Geometry check sheet. Reference: the model listing, model coordinates, mm. A direction names the side the tool comes from. Round coordinates to 2 decimals unless told otherwise and drop trailing zeros. Order: outer loops, then holes, each group sorted by start corner. A loop starts at its lowest first (then second) coordinate and runs counter-clockwise, first axis right, second up. Notation, with made-up numbers: (43, 52) -> (58, 52) arc R12 cw to (58, 64) -> close; hole circle Ø4 at (-1, 63). An arc over 180 degrees is marked (long way). Use a Markdown table: item, result. Add a question column.
Item 1: Sectioned sample at C-C, the plane z = 47. Record the cut outline in (x, y), and give its area (3 significant figures).
Item 2: Gauge pin test, flat ends, axial feed: pin 1 Ø4 at (x, z) = (-16.5, 75) entering from -Y; pin 2 Ø0.6 at (y, z) = (12.5, 202) entering from +X; pin 3 Ø10.5 at (y, z) = (19.5, 99) entering from +X; pin 4 Ø1.3 at (y, z) = (22.5, -2.5) entering from -X. Record the tip position at first contact, or that the pin passes through.
Item 3: Set-up check for faces 1 (the flat face through (-31, 22.103, -2)), 2 (the flat face through (-61.179, 17, 108)), 3 (the flat face through (-61, 23.303, 75)), 4 (the flat face through (-39, 1, 220)), 5 (the flat face through (-30, 13, 2)): record each of +Z, -Z, +X, -X, +Y, -Y from which the full face is reachable in a straight line by a thin tool's end or side.
Item 4: Sectioned sample at D-D, the plane y = 9. Record the cut outline in (x, z).
Item 5: Sectioned sample at B-B, the plane x = -35. Record the cut outline in (y, z), and give its area (3 significant figures).
Item 6: Material ranges on probe 1 along X at (y, z) = (13.5, 34.5); probe 2 along X at (y, z) = (21.75, 135.5); probe 3 along Z at (x, y) = (-13.5, 21.5), recorded low to high. Write a range as [from, to].
Item 7: Sectioned sample at A-A, the plane z = 149. Record the cut outline in (x, y).
from build123d import *

# Parameters (mm, degrees)
F1_DEPTH = 220
F3_DEPTH = 2
F5_DEPTH = 2
F6_W     = 61.179483
F6_H     = 1.2
F7_DEPTH = 5


with BuildPart() as f1:
    # F0 (on Top) → F1 (new body)
    with BuildSketch(Plane.XY):
        Polygon((-51.641022, 0), (0, 0), (0, 2), (-49.641022, 2), (-49.641022, 13.641025), (-59.179483, 13.641025), (-59.179483, 23.302566), (-63.948719, 23.302566), (-63.948719, 22.102566), (-61.179483, 22.102566), (-61.179483, 11.641025), (-51.641022, 11.641025), align=None)
    extrude(amount=F1_DEPTH)

    # F2 (on face) → F3 (cut, through all)
    with BuildSketch(Plane(origin=(0, 13.641025, 0), x_dir=(-1, 0, 0), z_dir=(0, 1, 0))):
        with BuildLine():
            Line((57.179483, 189.76923), (57.179483, 214.23077))
            ThreePointArc((57.179483, 214.23077), (54.410253, 217), (51.641022, 214.23077))
            Line((51.641022, 214.23077), (51.641022, 189.76923))
            ThreePointArc((51.641022, 189.76923), (54.410253, 187), (57.179483, 189.76923))
        make_face()
        with BuildLine():
            Line((57.179483, 144.76923), (57.179483, 169.23077))
            ThreePointArc((57.179483, 169.23077), (54.410253, 172), (51.641022, 169.23077))
            Line((51.641022, 169.23077), (51.641022, 144.76923))
            ThreePointArc((51.641022, 144.76923), (54.410253, 142), (57.179483, 144.76923))
        make_face()
        with BuildLine():
            Line((57.179483, 99.76923), (57.179483, 124.23077))
            ThreePointArc((57.179483, 124.23077), (54.410253, 127), (51.641022, 124.23077))
            Line((51.641022, 124.23077), (51.641022, 99.76923))
            ThreePointArc((51.641022, 99.76923), (54.410253, 97), (57.179483, 99.76923))
        make_face()
        with BuildLine():
            Line((57.179483, 54.76923), (57.179483, 79.23077))
            ThreePointArc((57.179483, 79.23077), (54.410253, 82), (51.641022, 79.23077))
            Line((51.641022, 79.23077), (51.641022, 54.76923))
            ThreePointArc((51.641022, 54.76923), (54.410253, 52), (57.179483, 54.76923))
        make_face()
        with BuildLine():
            Line((57.179483, 9.76923), (57.179483, 34.23077))
            ThreePointArc((57.179483, 34.23077), (54.410253, 37), (51.641022, 34.23077))
            Line((51.641022, 34.23077), (51.641022, 9.76923))
            ThreePointArc((51.641022, 9.76923), (54.410253, 7), (57.179483, 9.76923))
        make_face()
    extrude(amount=-F3_DEPTH, mode=Mode.SUBTRACT)

    # F4 (on face) → F5 (join)
    with BuildSketch(Plane(origin=(0, 0, 0), x_dir=(1, 0, 0), z_dir=(0, 0, -1))):
        Polygon((-59.179483, -13.641025), (-59.179483, -23.302566), (0, -23.302566), (0, -2), (-49.641022, -2), (-49.641022, -13.641025), align=None)
    extrude(amount=-F5_DEPTH)

    # F6 (on face) → F7 (join)
    with BuildSketch(Plane(origin=(0, 0, 0), x_dir=(1, 0, 0), z_dir=(0, 0, -1))):
        with Locations((-30.589741, -22.702566)):
            Rectangle(F6_W, F6_H)
    extrude(amount=F7_DEPTH)


solid = f1.part
Found:
| question | item | result |
|---|---|---|
| 1 | outline | (-63.95, 22.1) -> (-61.18, 22.1) -> (-61.18, 11.64) -> (-51.64, 11.64) -> (-51.64, 0) -> (0, 0) -> (0, 2) -> (-49.64, 2) -> (-49.64, 13.64) -> (-59.18, 13.64) -> (-59.18, 23.3) -> (-63.95, 23.3) -> close |
| 1 | area | 168 mm2 |
| 2 | pin 1 | stops at y = 0 |
| 2 | pin 2 | stops at x = -49.64 |
| 2 | pin 3 | stops at x = -59.18 |
| 2 | pin 4 | stops at x = -61.18 |
| 3 | face 1 | -Z, +X, -X, -Y |
| 3 | face 2 | +Z, -Z, -X, -Y |
| 3 | face 3 | +Z, -Z, +X, -X, +Y |
| 3 | face 4 | +Z, +X, -X, +Y, -Y |
| 3 | face 5 | +Z, +X, +Y |
| 4 | outline | (-51.64, 0) -> (0, 0) -> (0, 2) -> (-49.64, 2) -> (-49.64, 220) -> (-51.64, 220) -> close |
| 5 | outline | (0, 0) -> (22.1, 0) -> (22.1, -5) -> (23.3, -5) -> (23.3, 2) -> (2, 2) -> (2, 220) -> (0, 220) -> close |
| 5 | area | 489 mm2 |
| 6 | probe 1 | x = [-61.18, -57.17], [-51.65, -49.64] |
| 6 | probe 2 | x = [-61.18, -59.18] |
| 6 | probe 3 | z = [0, 2] |
| 7 | outline | (-63.95, 22.1) -> (-61.18, 22.1) -> (-61.18, 11.64) -> (-57.18, 11.64) -> (-57.18, 13.64) -> (-59.18, 13.64) -> (-59.18, 23.3) -> (-63.95, 23.3) -> close; (-51.64, 0) -> (0, 0) -> (0, 2) -> (-49.64, 2) -> (-49.64, 13.64) -> (-51.64, 13.64) -> close |
